```python
from build123d import *

# Parameters (mm, degrees)
SKETCH1_R                  = 3
EXTRUDE2_DEPTH             = 2
SKETCHED_START             = 1.456569183
SKETCHED_BEND1_OUTLINE_W   = 2
SKETCHED_BEND1_OUTLINE_H   = 30
SKETCHED_BEND1_DEPTH       = 28.543430817
SKETCHED_START_2           = 0.073009183
SKETCHED_BEND1_2_OUTLINE_R = 3
SKETCHED_BEND1_2_DEPTH     = 0.036590817
SKETCHED_START_3           = 0.608704599
SKETCHED_BEND1_3_OUTLINE_W = 2
SKETCHED_BEND1_3_OUTLINE_H = 30
SKETCHED_BEND1_3_DEPTH     = 0.847864584
SKETCHED_START_4           = -3.926990817
SKETCHED_BEND1_4_OUTLINE_R = 3
SKETCHED_BEND1_4_DEPTH     = 6
SKETCHED_START_5           = -15
SKETCHED_BEND1_5_DEPTH     = 30


with BuildPart() as part:
    # Sketch1 → Extrude2 (new body)
    with BuildSketch(Plane(origin=(0, 0, 0), x_dir=(1, 0, 0), z_dir=(0, 1, 0))):
        with BuildLine():
            Line((-20, -15), (20, -15))
            ThreePointArc((20, -15), (27.071067812, -12.071067812), (30, -5))
            Line((30, -5), (30, 5))
            ThreePointArc((30, 5), (27.071067812, 12.071067812), (20, 15))
            Line((20, 15), (-20, 15))
            ThreePointArc((-20, 15), (-27.071067812, 12.071067812), (-30, 5))
            Line((-30, 5), (-30, -5))
            ThreePointArc((-30, -5), (-27.071067812, -12.071067812), (-20, -15))
        make_face()
        with Locations(Location((-17.5, 0, 0), (0, 0, 270))):
            Circle(SKETCH1_R, mode=Mode.SUBTRACT)
        with Locations(Location((17.5, 0, 0), (0, 0, 90))):
            Circle(SKETCH1_R, mode=Mode.SUBTRACT)
    extrude(amount=EXTRUDE2_DEPTH)

    # Sketched Bend1: read off the stored shape, not the designer's step
    # Sketched Bend1 outline → Sketched Bend1 (cut)
    with BuildSketch(Plane.YZ.offset(SKETCHED_START)):
        with Locations((1, 0)):
            Rectangle(SKETCHED_BEND1_OUTLINE_W, SKETCHED_BEND1_OUTLINE_H)
    extrude(amount=SKETCHED_BEND1_DEPTH, mode=Mode.SUBTRACT)

    # Sketched Bend1 2 outline → Sketched Bend1 2 (add)
    with BuildSketch(Plane.YZ.offset(SKETCHED_START_2)):
        with BuildLine():
            Line((22.073009183, 15), (2, 15))
            Line((2, 15), (2, -15))
            Line((2, -15), (22.073009183, -15))
            ThreePointArc((22.073009183, -15), (29.144076995, -12.071067812), (32.073009183, -5))
            Line((32.073009183, -5), (32.073009183, 5))
            ThreePointArc((32.073009183, 5), (29.144076995, 12.071067812), (22.073009183, 15))
        make_face()
        with Locations((19.573009183, 0)):
            Circle(SKETCHED_BEND1_2_OUTLINE_R, mode=Mode.SUBTRACT)
    extrude(amount=SKETCHED_BEND1_2_DEPTH)

    # Sketched Bend1 3 outline → Sketched Bend1 3 (cut)
    with BuildSketch(Plane.YZ.offset(SKETCHED_START_3)):
        with Locations((1, 0)):
            Rectangle(SKETCHED_BEND1_3_OUTLINE_W, SKETCHED_BEND1_3_OUTLINE_H)
    extrude(amount=SKETCHED_BEND1_3_DEPTH, mode=Mode.SUBTRACT)

    # Sketched Bend1 4 outline → Sketched Bend1 4 (add)
    with BuildSketch(Plane.YZ.offset(SKETCHED_START_4)):
        with BuildLine():
            Line((22.073009183, 15), (2, 15))
            Line((2, 15), (2, -15))
            Line((2, -15), (22.073009183, -15))
            ThreePointArc((22.073009183, -15), (29.144076995, -12.071067812), (32.073009183, -5))
            Line((32.073009183, -5), (32.073009183, 5))
            ThreePointArc((32.073009183, 5), (29.144076995, 12.071067812), (22.073009183, 15))
        make_face()
        with Locations((19.573009183, 0)):
            Circle(SKETCHED_BEND1_4_OUTLINE_R, mode=Mode.SUBTRACT)
    extrude(amount=SKETCHED_BEND1_4_DEPTH)

    # Sketched Bend1 5 outline → Sketched Bend1 5 (cut)
    with BuildSketch(Plane.XY.offset(SKETCHED_START_5)):
        with BuildLine():
            ThreePointArc((-3.926990817, 2), (-1.098563692, 3.171572875), (0.073009183, 6))
            Line((0.073009183, 6), (0.073009183, 32.073009183))
            Line((0.073009183, 32.073009183), (-3.926990817, 32.073009183))
            Line((-3.926990817, 32.073009183), (-3.926990817, 2))
        make_face()
        with BuildLine():
            Line((2.073009183, 2), (2.073009183, 6))
            ThreePointArc((2.073009183, 6), (0.31564987, 1.757359313), (-3.926990817, 0))
            Line((-3.926990817, 0), (0.608704599, 0))
            Line((0.608704599, 0), (0.608704599, 2))
            Line((0.608704599, 2), (2.073009183, 2))
        make_face()
    extrude(amount=SKETCHED_BEND1_5_DEPTH, mode=Mode.SUBTRACT)


solid = part.part
```
Geometry: final body of the model. Coordinates: model frame, mm. A direction names the side the tool comes from. Give positions to 0.01 mm unless a question says otherwise; leave off trailing zeros. Loops run counter-clockwise (first coordinate to the right, second up) from the corner with the lowest first, then second, coordinate; pieces in that order, holes last. Notation, with made-up numbers: (4.25, 31) - (55.25, 31) arc R29 cw to (55.25, 51) - close; hole circle Ø7 at (-5, -4.75). An arc over 180 degrees is marked (long way). Answer as CSV lines item,"result". Start each with the question number.
(1) Mould query, pull axis X, two halves, no side actions, for faces 1 (the face through (-26.99, 0.99, -12.15)), 2 (the face through (1.059, 29.221, 11.993)), 3 (the face through (-20.43, 0.99, -0.65)). Classes: +X half, -X half, draft (parallel to the pull), parting line (faces both ways), or undercut.
(2) Section query C-C (z = 10). Output: boundary loops of the cut face in (x, y), and give its area (3 significant figures).
(3) Section query B-B (x = -17.5). Output: boundary loops of the cut face in (y, z).
(4) Section query D-D (y = 12.5). Output: boundary loops of the cut face in (x, z).
(5) Pin query (flat end, axial travel): P1, Ø2, axis at x = -22.5, z = -1.5, coming from the -Y side; P2, Ø5.5, axis at y = 19.57, z = 0, coming from the +X side; P3, Ø4, axis at x = -22.5, z = 11, coming from the +Y side; P4, Ø5, axis at y = 12.5, z = 0.5, coming from the -X side. Return the tip coordinate at first contact, or that it passes through.
(6) Reachability of faces 4 (the face through (-14, 2, 0)), 5 (the face through (2.073, 16, 0)) from +Z, -Z, +X, -X, +Y, -Y: full face, straight path, thin tool, end or side. Return the list, or none.
(7) Ray query, line 1 along X through (y, z) = (7.5, 10.5); line 2 along Y through (x, z) = (-21, -11.5); line 3 along X through (y, z) = (1, 0). Return the intervals inside material, ascending. Write a range as [from, to].
(8) Section query A-A (z = 0). Output: boundary loops of the cut face in (x, y), and give its area (3 significant figures).
Worked answers:
1,face 1,"-X half"
1,face 2,"draft"
1,face 3,"undercut"
2,outline,"(-28.66, 0) - (-3.93, 0) arc R6 ccw to (2.07, 6) - (2.07, 30.73) - (0.07, 30.73) - (0.07, 6) arc R4 cw to (-3.93, 2) - (-28.66, 2) - close"
2,area,"115 mm^2"
3,outline,"(0, -15) - (2, -15) - (2, -3) - (0, -3) - close; (0, 3) - (2, 3) - (2, 15) - (0, 15) - close"
4,outline,"(0.07, -15) - (2.07, -15) - (2.07, 15) - (0.07, 15) - close"
5,P1,"stops at y = 0"
5,P2,"passes through"
5,P3,"stops at y = 2"
5,P4,"stops at x = 0.07"
6,face 4,"+Z, -Z, -X, +Y"
6,face 5,"+Z, -Z, +X, +Y, -Y"
7,line 1,"x = [0.07, 2.07]"
7,line 2,"y = [0, 2]"
7,line 3,"x = [-30, -20.5], [-14.5, -0.61]"
8,outline,"(-30, 0) - (-20.5, 0) - (-20.5, 2) - (-30, 2) - close; (-14.5, 0) - (-3.93, 0) arc R6 ccw to (2.07, 6) - (2.07, 16.57) - (0.07, 16.57) - (0.07, 6) arc R4 cw to (-3.93, 2) - (-14.5, 2) - close; (0.07, 22.57) - (2.07, 22.57) - (2.07, 32.07) - (0.07, 32.07) - close"
8,area,"96.0 mm^2"
